from build123d import *

# Parameters (mm, degrees)
SKETCH2_W            = 30
SKETCH2_H            = 20
BOSS_EXTRUDE1_DEPTH  = 15
CUT_EXTRUDE1_DEPTH   = 18.2
SKETCH4_W            = 2.5
SKETCH4_H            = 0.5
BOSS_EXTRUDE2_DEPTH  = 3
FILLET1_R            = 1.5
FILLET1_OF_MIRROR2_R = 1.5
FILLET2_R            = 1.5


with BuildPart() as part:
    # Sketch2 → Boss-Extrude1 (new body)
    with BuildSketch(Plane(origin=(0, 0, 0), x_dir=(1, 0, 0), z_dir=(0, 1, 0))):
        Rectangle(SKETCH2_W, SKETCH2_H)
    extrude(amount=BOSS_EXTRUDE1_DEPTH)

    # Sketch3 → Cut-Extrude1 (cut)
    with BuildSketch(Plane.XY.offset(10)):
        Polygon((-11.2, 15), (-11.2, 6.45), (-1.8, 6.45), (-1.8, 11.25), (-4.8, 11.25), (-4.8, 15), align=None)
    cut_extrude1 = extrude(amount=-CUT_EXTRUDE1_DEPTH, mode=Mode.SUBTRACT)

    # Sketch4 → Boss-Extrude2 (add)
    with BuildSketch(Plane.ZY.offset(1.8)):
        with Locations((5.85, 11)):
            Rectangle(SKETCH4_W, SKETCH4_H)
        with Locations((-2.15, 11)):
            Rectangle(SKETCH4_W, SKETCH4_H)
    boss_extrude2 = extrude(amount=BOSS_EXTRUDE2_DEPTH)

    # Fillet1
    # the kernel refuses this fillet: 1.5 mm, written as the material it takes off along each edge
    with BuildSketch(Plane(origin=(-1.8, 10.75, 4.6), x_dir=(0, 0, 1), z_dir=(-1, 0, 0)), Plane(origin=(-1.8, 10.75, -3.4), x_dir=(0, 0, 1), z_dir=(-1, 0, 0))) as fillet1_piece_1:
        with BuildLine():
            CenterArc((1.118033989, 1.5), FILLET1_R, 221.810314896, 48.189685104)
            Line((0, 0.5), (-0.02236068, 0.48))
            ThreePointArc((-0.02236068, 0.48), (-0.03, 0.25), (-0.03, 0))
            Line((-0.03, 0), (0, -0.03))
            Line((0, -0.03), (1.118033989, -0.03))
            Line((1.118033989, -0.03), (1.118033989, 0))
        make_face()
    extrude(amount=5.795084972, mode=Mode.SUBTRACT)
    with BuildSketch(Plane(origin=(-1.8, 10.75, 7.1), x_dir=(0, 1, 0), z_dir=(-1, 0, 0)), Plane(origin=(-1.8, 10.75, -0.9), x_dir=(0, 1, 0), z_dir=(-1, 0, 0))) as fillet1_piece_2:
        with BuildLine():
            CenterArc((1.5, 1.118033989), FILLET1_R, 180, 48.189685104)
            Line((0, 1.118033989), (-0.03, 1.118033989))
            Line((-0.03, 1.118033989), (-0.03, 0))
            Line((-0.03, 0), (0, -0.03))
            ThreePointArc((0, -0.03), (0.25, -0.03), (0.48, -0.02236068))
            Line((0.48, -0.02236068), (0.5, 0))
        make_face()
    extrude(amount=5.795084972, mode=Mode.SUBTRACT)

    # Mirror2: Cut-Extrude1, Boss-Extrude2 across plane
    add(cut_extrude1.mirror(Plane(origin=(0, 0, 0), x_dir=(0, 0, 1), z_dir=(1, 0, 0))), mode=Mode.SUBTRACT)
    add(boss_extrude2.mirror(Plane(origin=(0, 0, 0), x_dir=(0, 0, 1), z_dir=(1, 0, 0))))

    # Fillet1 of Mirror2
    # the kernel refuses this fillet: 1.5 mm, written as the material it takes off along each edge
    with BuildSketch(Plane(origin=(1.8, 10.75, 4.6), x_dir=(0, 0, 1), z_dir=(1, 0, 0)), Plane(origin=(1.8, 10.75, -3.4), x_dir=(0, 0, 1), z_dir=(1, 0, 0))) as fillet1_of_mirror2_piece_1:
        with BuildLine():
            CenterArc((1.118033989, -1.5), FILLET1_OF_MIRROR2_R, 90, 48.189685104)
            Line((0, -0.5), (-0.02236068, -0.48))
            ThreePointArc((-0.02236068, -0.48), (-0.03, -0.25), (-0.03, 0))
            Line((-0.03, 0), (0, 0.03))
            Line((0, 0.03), (1.118033989, 0.03))
            Line((1.118033989, 0.03), (1.118033989, 0))
        make_face()
    extrude(amount=5.795084972, mode=Mode.SUBTRACT)
    with BuildSketch(Plane(origin=(1.8, 10.75, 7.1), x_dir=(0, 1, 0), z_dir=(1, 0, 0)), Plane(origin=(1.8, 10.75, -0.9), x_dir=(0, 1, 0), z_dir=(1, 0, 0))) as fillet1_of_mirror2_piece_2:
        with BuildLine():
            CenterArc((1.5, -1.118033989), FILLET1_OF_MIRROR2_R, 131.810314896, 48.189685104)
            Line((0, -1.118033989), (-0.03, -1.118033989))
            Line((-0.03, -1.118033989), (-0.03, 0))
            Line((-0.03, 0), (0, 0.03))
            ThreePointArc((0, 0.03), (0.25, 0.03), (0.48, 0.02236068))
            Line((0.48, 0.02236068), (0.5, 0))
        make_face()
    extrude(amount=5.795084972, mode=Mode.SUBTRACT)

    # Fillet2
    fillet2_edges = [part.edges().sort_by_distance(p)[0] for p in [
        (0, 0, 10),
        (-15, 0, 0),
        (0, 0, -10),
        (15, 0, 0),
        (15, 7.5, 10),
        (-15, 7.5, 10),
        (-15, 7.5, -10),
        (15, 7.5, -10),
    ]]
    fillet(fillet2_edges, radius=FILLET2_R)


solid = part.part
Work out the finished part from the listing and answer in its coordinate system (mm). A direction names the side the tool comes from. Coordinates: 2 decimals unless noted, no trailing zeros. Loops run counter-clockwise (first coordinate to the right, second up) from the corner with the lowest first, then second, coordinate; pieces in that order, holes last. Notation, with made-up numbers: (-37, -39.5) -> (-24, -39.5) arc R21 cw to (-24, -8.5) -> close; hole circle Ø3 at (22.5, 54). An arc over 180 degrees is marked (long way). Answer as CSV lines item,"result".
1) The part is cut by section D-D (y = 8.5). Give the vertices of the cut face in (x, z).
A:
outline,"(-15, -8.5) arc R1.5 ccw to (-13.5, -10) -> (13.5, -10) arc R1.5 ccw to (15, -8.5) -> (15, 8.5) arc R1.5 ccw to (13.5, 10) -> (11.2, 10) -> (11.2, -8.2) -> (1.8, -8.2) -> (1.8, 10) -> (-1.8, 10) -> (-1.8, -8.2) -> (-11.2, -8.2) -> (-11.2, 10) -> (-13.5, 10) arc R1.5 ccw to (-15, 8.5) -> close"
2) Straight lines are drawn through the part: probe 1 along X at (y, z) = (12.25, 7.75); probe 2 along X at (y, z) = (10.5, 4); probe 3 along Y at (x, z) = (-4, 1.75). For each, find the intervals that lie inside material, in ascending order.
A:
probe 1,"x = -15 to -11.2, -4.8 to 4.8, 11.2 to 15"
probe 2,"x = -15 to -11.2, -1.8 to 1.8, 11.2 to 15"
probe 3,"y = 0 to 6.45, 11.25 to 15"
3) For a pull along X with two mould halves and no side action, classify faces 1 (the face through (0.19, 0.45, -9.57)), 2 (the face through (14.55, 8.34, 9.57)), 3 (the face through (3.279, 10.884, 6.602)) as released by +X, released by -X, zero draft, split by the parting line, or undercut.
A:
face 1,"zero draft"
face 2,"released by +X"
face 3,"undercut"
4) Flat-ended cylindrical pins translate along their axes: pin 1 (2.5 mm diameter, centred on x = -8, y = 9, fed in from +Z); pin 2 (3 mm diameter, centred on x = 10.5, z = -1, fed in from +Y). Find the tip coordinate at first contact, or state that the pin passes through.
A:
pin 1,"stops at z = -8.2"
pin 2,"stops at y = 15"
5) The part is cut by section B-B (x = 8.25). Give the vertices of the cut face in (y, z).
A:
outline,"(0, -8.5) arc R1.5 ccw to (1.5, -10) -> (15, -10) -> (15, -8.2) -> (6.45, -8.2) -> (6.45, 10) -> (1.5, 10) arc R1.5 ccw to (0, 8.5) -> close"
6) The part is cut by section A-A (y = 12). Give the vertices of the cut face in (x, z), and give its area (3 significant figures).
A:
outline,"(-15, -8.5) arc R1.5 ccw to (-13.5, -10) -> (13.5, -10) arc R1.5 ccw to (15, -8.5) -> (15, 8.5) arc R1.5 ccw to (13.5, 10) -> (11.2, 10) -> (11.2, -8.2) -> (4.8, -8.2) -> (4.8, 10) -> (-4.8, 10) -> (-4.8, -8.2) -> (-11.2, -8.2) -> (-11.2, 10) -> (-13.5, 10) arc R1.5 ccw to (-15, 8.5) -> close"
area,"365 mm²"
7) For faces 4 (the face through (-3.28, 10.88, 6.59)), 5 (the face through (3, 11.25, 2)), 6 (the face through (4.8, 13, 1)), determine the directions among +Z, -Z, +X, -X, +Y, -Y from which every point of the face is accessible in a straight line to the end or side of a thin tool.
A:
face 4,"+Z"
face 5,"none"
face 6,"+Z, +Y"
8) The part is cut by section C-C (z = -6.25). Give the vertices of the cut face in (x, y).
A:
outline,"(-15, 1.5) arc R1.5 ccw to (-13.5, 0) -> (13.5, 0) arc R1.5 ccw to (15, 1.5) -> (15, 15) -> (11.2, 15) -> (11.2, 6.45) -> (1.8, 6.45) -> (1.8, 11.25) -> (4.8, 11.25) -> (4.8, 15) -> (-4.8, 15) -> (-4.8, 11.25) -> (-1.8, 11.25) -> (-1.8, 6.45) -> (-11.2, 6.45) -> (-11.2, 15) -> (-15, 15) -> close"
